Check sheet for the drawn part. Datum: minimum x, y, z corner. Units: mm. Round coordinates to 2 decimals unless told otherwise and drop trailing zeros. Write each loop counter-clockwise with the first axis right and the second up, starting at its lowest first coordinate (ties: lowest second). Pieces come first, ordered by that corner, then holes. Notation, with made-up numbers: (-12, 18.25) -> (29, 18.25) arc R28 cw to (29, 46.25) -> close; hole circle Ø5 at (66.25, -14.75). An arc over 180 degrees is marked (long way). Use a Markdown table: item, result.
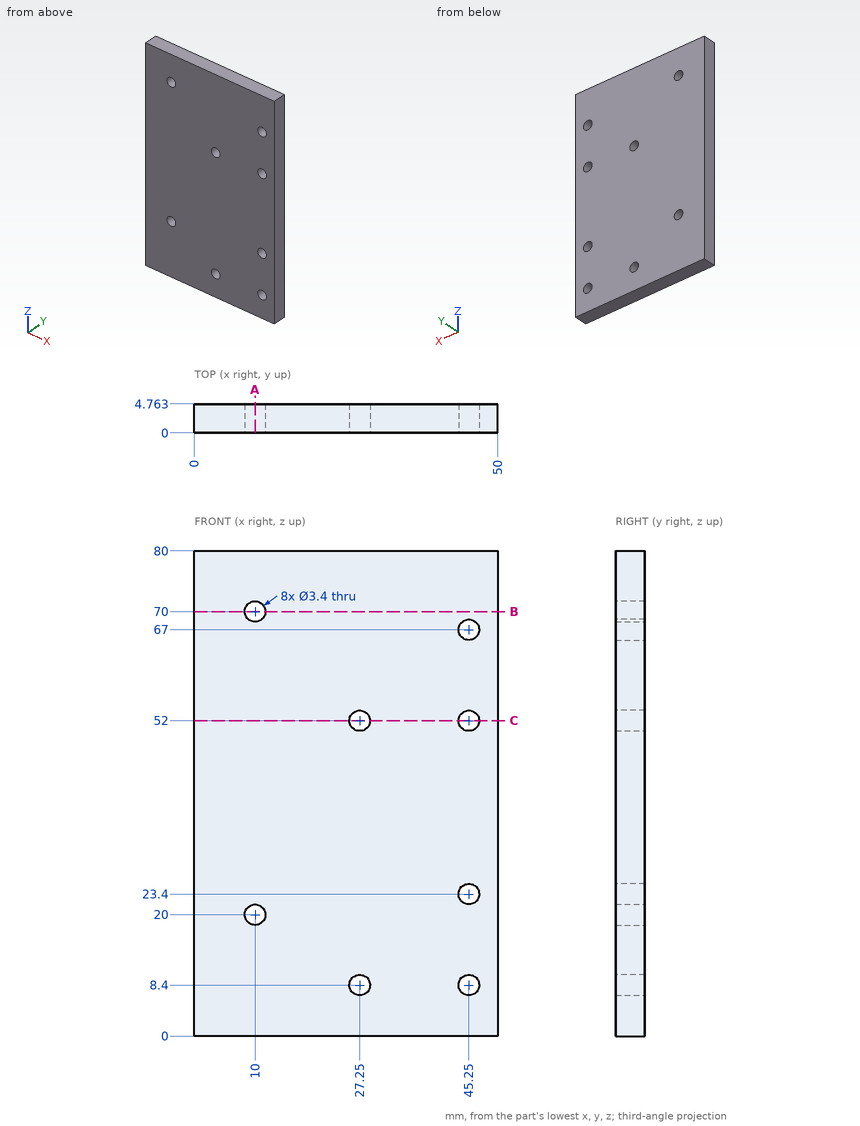
(1) Gauge pin test, flat end, axial feed: pin 1 Ø3 at (x, z) = (10, 20) entering from -Y. Record the tip position at first contact, or that the pin passes through.
A:
| item | result |
|---|---|
| pin 1 | passes through |
(2) Section check B-B on z = 70. Record the cut outline in (x, y), plus the area to 3 significant figures.
A:
| item | result |
|---|---|
| outline | (0, 0) -> (8.3, 0) -> (8.3, 4.76) -> (0, 4.76) -> close; (11.7, 0) -> (50, 0) -> (50, 4.76) -> (11.7, 4.76) -> close |
| area | 222 mm2 |
(3) Thickness scan on line 1 (Z direction, x = 45.25, y = 2.9); line 2 (X direction, y = 2.1, z = 8.4); line 3 (Z direction, x = 9, y = 0.75) (1 decimal). Record the ranges inside material, lowest first.
A:
| item | result |
|---|---|
| line 1 | z = 0 to 6.7, 10.1 to 21.7, 25.1 to 50.3, 53.7 to 65.3, 68.7 to 80 |
| line 2 | x = 0 to 25.55, 28.95 to 43.55, 46.95 to 50 |
| line 3 | z = 0 to 18.6, 21.4 to 68.6, 71.4 to 80 |
(4) Section check C-C on z = 52. Record the cut outline in (x, y).
A:
| item | result |
|---|---|
| outline | (0, 0) -> (25.55, 0) -> (25.55, 4.76) -> (0, 4.76) -> close; (28.95, 0) -> (43.55, 0) -> (43.55, 4.76) -> (28.95, 4.76) -> close; (46.95, 0) -> (50, 0) -> (50, 4.76) -> (46.95, 4.76) -> close |
(5) Section check A-A on x = 10. Record the cut outline in (y, z).
A:
| item | result |
|---|---|
| outline | (0, 0) -> (4.76, 0) -> (4.76, 18.3) -> (0, 18.3) -> close; (0, 21.7) -> (4.76, 21.7) -> (4.76, 68.3) -> (0, 68.3) -> close; (0, 71.7) -> (4.76, 71.7) -> (4.76, 80) -> (0, 80) -> close |
